Check sheet for the modelled part. Datum: model origin and axes. Units: mm. A direction names the side the tool comes from. Give positions to 0.01 mm unless a question says otherwise; leave off trailing zeros.
Item 1: Release check for a two-part mould opening along X. For faces 1 (the flat face through (0, -10, -50.038)), 2 (the flat face through (-14.887, -10, 45)) record: released by +X, released by -X, zero draft, split by the parting line, or undercut.
Item 2: Sectioned sample at A-A on y = -18. Count the separate pieces of the cut face and the enclosed holes in it, and give its area (3 significant figures).
Item 3: Material ranges on line 1 along Z through (x, y) = (-12, -6.5); line 2 along Z through (x, y) = (-3, -18), recorded low to high.
Item 4: Access from +Z, -Z, +X, -X, +Y, -Y to the whole of each face (thin tool, end or side, straight path). Record for faces 3 (the flat face through (1, -10, 42.034)), 4 (the flat face through (0, -10, 50.038)).
from build123d import *

# Parameters (mm, degrees)
F0_W     = 45.974
F0_H     = 100.076
F1_DEPTH = 21.082


with BuildPart() as f1:
    # F0 (on Front) → F1 (new body)
    with BuildSketch(Plane.XZ):
        Rectangle(F0_W, F0_H)
        with BuildLine():
            Line((-17.7857931137, 44.2633313295), (-18.9050379284, 44.2633313295))
            Line((-18.9050379284, 44.2633313295), (-18.9050379284, 42.034227401))
            Line((-18.9050379284, 42.034227401), (-19.5280138157, 42.034227401))
            Line((-19.5280138157, 42.034227401), (-19.5280138157, 47.3946357427))
            Line((-19.5280138157, 47.3946357427), (-18.0579784355, 47.3946357427))
            add(Edge.make_bspline(
                [(-18.0579784355, 47.3946357427), (-17.071306644, 47.3946357427), (-16.6002617876, 47.0168612875)],
                knots=[0, 0, 0, 1, 1, 1], degree=2))
            add(Edge.make_bspline(
                [(-16.6002617876, 47.0168612875), (-16.1292169311, 46.6390868322), (-16.1292169311, 45.8800182839)],
                knots=[0, 0, 0, 1, 1, 1], degree=2))
            add(Edge.make_bspline(
                [(-16.1292169311, 45.8800182839), (-16.1292169311, 44.8170876738), (-17.2073993049, 44.4428328564)],
                knots=[0, 0, 0, 1, 1, 1], degree=2))
            Line((-17.2073993049, 44.4428328564), (-15.7514424759, 42.034227401))
            Line((-15.7514424759, 42.034227401), (-16.4882199848, 42.034227401))
            Line((-16.4882199848, 42.034227401), (-17.7857931137, 44.2633313295))
        make_face(mode=Mode.SUBTRACT)
        Polygon((-11.8986123174, 42.5915033831), (-11.8986123174, 42.034227401), (-14.8867847941, 42.034227401), (-14.8867847941, 47.3946357427), (-11.8986123174, 47.3946357427), (-11.8986123174, 46.8408793984), (-14.2638089067, 46.8408793984), (-14.2638089067, 45.1139104601), (-12.0417442538, 45.1139104601), (-12.0417442538, 44.5636737536), (-14.2638089067, 44.5636737536), (-14.2638089067, 42.5915033831), align=None, mode=Mode.SUBTRACT)
        Polygon((-6.6965876758, 42.034227401), (-7.3418546025, 42.034227401), (-8.0094125685, 43.7389053), (-10.157564828, 43.7389053), (-10.8169103057, 42.034227401), (-11.4480986813, 42.034227401), (-9.3292767366, 47.416926782), (-8.8048507071, 47.416926782), align=None, mode=Mode.SUBTRACT)
        with BuildLine():
            add(Edge.make_bspline(
                [(-2.3738858735, 46.701853706), (-1.6811038367, 46.0090716693), (-1.6811038367, 44.7654663197)],
                knots=[0, 0, 0, 1, 1, 1], degree=2))
            add(Edge.make_bspline(
                [(-1.6811038367, 44.7654663197), (-1.6811038367, 43.438562876), (-2.4014563694, 42.7363951385)],
                knots=[0, 0, 0, 1, 1, 1], degree=2))
            add(Edge.make_bspline(
                [(-2.4014563694, 42.7363951385), (-3.1218089021, 42.034227401), (-4.4745230229, 42.034227401)],
                knots=[0, 0, 0, 1, 1, 1], degree=2))
            Line((-4.4745230229, 42.034227401), (-5.9598101668, 42.034227401))
            Line((-5.9598101668, 42.034227401), (-5.9598101668, 47.3946357427))
            Line((-5.9598101668, 47.3946357427), (-4.3173125353, 47.3946357427))
            add(Edge.make_bspline(
                [(-4.3173125353, 47.3946357427), (-3.0666679102, 47.3946357427), (-2.3738858735, 46.701853706)],
                knots=[0, 0, 0, 1, 1, 1], degree=2))
        make_face(mode=Mode.SUBTRACT)
        Polygon((2.5025722732, 42.5915033831), (2.5025722732, 42.034227401), (-0.4856002035, 42.034227401), (-0.4856002035, 47.3946357427), (2.5025722732, 47.3946357427), (2.5025722732, 46.8408793984), (0.1373756839, 46.8408793984), (0.1373756839, 45.1139104601), (2.3594403368, 45.1139104601), (2.3594403368, 44.5636737536), (0.1373756839, 44.5636737536), (0.1373756839, 42.5915033831), align=None, mode=Mode.SUBTRACT)
        with BuildLine():
            Line((5.4320841203, 44.2633313295), (4.3128393057, 44.2633313295))
            Line((4.3128393057, 44.2633313295), (4.3128393057, 42.034227401))
            Line((4.3128393057, 42.034227401), (3.6898634183, 42.034227401))
            Line((3.6898634183, 42.034227401), (3.6898634183, 47.3946357427))
            Line((3.6898634183, 47.3946357427), (5.1598987985, 47.3946357427))
            add(Edge.make_bspline(
                [(5.1598987985, 47.3946357427), (6.14657059, 47.3946357427), (6.6176154465, 47.0168612875)],
                knots=[0, 0, 0, 1, 1, 1], degree=2))
            add(Edge.make_bspline(
                [(6.6176154465, 47.0168612875), (7.0886603029, 46.6390868322), (7.0886603029, 45.8800182839)],
                knots=[0, 0, 0, 1, 1, 1], degree=2))
            add(Edge.make_bspline(
                [(7.0886603029, 45.8800182839), (7.0886603029, 44.8170876738), (6.0104779291, 44.4428328564)],
                knots=[0, 0, 0, 1, 1, 1], degree=2))
            Line((6.0104779291, 44.4428328564), (7.4664347582, 42.034227401))
            Line((7.4664347582, 42.034227401), (6.7296572492, 42.034227401))
            Line((6.7296572492, 42.034227401), (5.4320841203, 44.2633313295))
        make_face(mode=Mode.SUBTRACT)
    extrude(amount=F1_DEPTH)


solid = f1.part
Report:
1. face 1: zero draft
1. face 2: undercut
2. separate pieces: 1
2. enclosed holes: 6
2. area: 4,530 mm2
3. line 1: z = -50.04 to 42.03, 42.59 to 46.84, 47.39 to 50.04
3. line 2: z = -50.04 to 42.32, 47.14 to 50.04
4. face 3: +Y, -Y
4. face 4: +Z, +X, -X, +Y, -Y
